from build123d import *

# Parameters (mm, degrees)
BOSS_EXTRUDE1_DEPTH      = 25.4
BOSS_EXTRUDE1_DEPTH_BACK = 25.4
FILLET1_R                = 19.05
SHELL1_T                 = -1.27
SKETCH4_R                = 5.5626
CUT_EXTRUDE1_DEPTH       = 50.947471892


with BuildPart() as part:
    # Sketch3 → Boss-Extrude1 (new body, two sides)
    with BuildSketch(Plane(origin=(0, 0, 0), x_dir=(0, 0, -1), z_dir=(1, 0, 0))) as boss_extrude1_sk:
        with BuildLine():
            Line((0, 39.37), (35.56, 39.37))
            ThreePointArc((35.56, 39.37), (107.217829782, 34.971995328), (177.8, 21.844))
            Line((177.8, 21.844), (177.8, -39.37))
            Line((177.8, -39.37), (0, -39.37))
            Line((0, -39.37), (0, 39.37))
        make_face()
    extrude(amount=BOSS_EXTRUDE1_DEPTH)
    extrude(boss_extrude1_sk.sketch, amount=-BOSS_EXTRUDE1_DEPTH_BACK)

    # Fillet1
    fillet1_edges = [part.edges().sort_by_distance(p)[0] for p in [
        (25.4, 34.971995328, -107.217829782),
        (-25.4, 39.37, -17.78),
        (-25.4, 34.971995328, -107.217829782),
        (25.4, 39.37, -17.78),
    ]]
    fillet(fillet1_edges, radius=FILLET1_R)

    # Shell1
    shell1_openings = [part.faces().sort_by_distance(p)[0] for p in [
        (0, -39.37, -88.9),
        (0, 8.088461394, 0),
    ]]
    offset(amount=SHELL1_T, openings=shell1_openings, kind=Kind.INTERSECTION)

    # Sketch4 → Cut-Extrude1 (cut)
    with BuildSketch(Plane(origin=(0, 0, -177.8), x_dir=(-1, 0, 0), z_dir=(0, 0, -1))):
        with Locations((0, -11.577471892)):
            Circle(SKETCH4_R)
    extrude(amount=-CUT_EXTRUDE1_DEPTH, mode=Mode.SUBTRACT)


solid = part.part
For this review, take the finished solid that the model builds, in its own axes (mm). A direction names the side the tool comes from. Round coordinates to 2 decimals unless told otherwise and drop trailing zeros. Loops run counter-clockwise (first coordinate to the right, second up) from the corner with the lowest first, then second, coordinate; pieces in that order, holes last. Notation, with made-up numbers: (-17, 84) - (18, 84) arc R33 cw to (18, 115) - close; hole circle Ø7 at (15.25, 87.25). An arc over 180 degrees is marked (long way). Use one line per item in the form item = value.
1) Clearance check with flat-ended pins moving along their axes: P1, Ø6.5, axis at x = 0, y = -11.58, coming from the -Z side; P2, Ø10, axis at x = -0.5, z = -22, coming from the -Y side; P3, Ø4, axis at y = 23, z = -37, coming from the -X side; P4, Ø12, axis at x = -13, z = -131.5, coming from the -Y side. State where each tip first meets the part, or that it passes through.
Solutions:
P1 = through
P2 = 38.1
P3 = -25.39
P4 = 24.73
2) We need section A-A on x = 0. Write out the cut boundary in (y, z), then the cut area to 3 significant figures.
Solutions:
outline = (-39.37, -177.8) - (-17.14, -177.8) - (-17.14, -176.53) - (-39.37, -176.53) - close; (-6.01, -177.8) - (21.84, -177.8) arc R585.97 ccw to (39.37, -35.56) - (39.37, 0) - (38.1, 0) - (38.1, -35.56) arc R584.7 cw to (20.85, -176.53) - (-6.01, -176.53) - close
area = 290 mm2
3) Wall thickness on probe 1 along X at (y, z) = (16, -48); probe 2 along Y at (x, z) = (5, -33.5); probe 3 along Z at (x, y) = (12, 6.5): over which ranges is each line inside the solid? List them lowest first.
Solutions:
probe_1 = -25.4 to -24.13, 24.13 to 25.4
probe_2 = 38.1 to 39.37
probe_3 = -177.8 to -176.53
4) Tool access review of faces 1 (the face through (0, 39.37, -18)), 2 (the face through (0.089, 33.892, -105.581)): name each direction out of +Z, -Z, +X, -X, +Y, -Y from which nothing blocks a thin tool from reaching the whole face with its end or side.
Solutions:
face_1 = +Z, -Z, +X, -X, +Y
face_2 = +Z, -Y
5) We need section B-B on y = -28.5. Write out the cut boundary in (x, z).
Solutions:
outline = (-25.4, -177.8) - (25.4, -177.8) - (25.4, 0) - (24.13, 0) - (24.13, -176.53) - (-24.13, -176.53) - (-24.13, 0) - (-25.4, 0) - close
6) We need section C-C on x = -11.5. Write out the cut boundary in (y, z).
Solutions:
outline = (-39.37, -177.8) - (21.11, -177.8) arc R585.26 ccw to (38.66, -35.56) - (38.66, 0) - (37.34, 0) - (37.34, -35.56) arc R583.94 cw to (20.07, -176.53) - (-39.37, -176.53) - close
